Can you work these out from the drawing? Everything is in mm from the part's minimum corner. A direction names the side the tool comes from. Round coordinates to 2 decimals unless told otherwise and drop trailing zeros. Write each loop counter-clockwise with the first axis right and the second up, starting at its lowest first coordinate (ties: lowest second). Pieces come first, ordered by that corner, then holes. Notation, with made-up numbers: (-8, 61.5) - (27, 61.5) arc R11 ccw to (27, 81.5) - close; hole circle Ø10 at (66.25, 86). An arc over 180 degrees is marked (long way). Write each question's results on one line, items separated by ' | '. Start each with the question number.
(1) Please list where these lines run through material, in increasing order: line 1 (X direction, y = 1, z = 15); line 2 (Z direction, x = 15, y = 4.75); line 3 (Z direction, x = 25, y = 0.55). Write a range as [from, to].
(2) Thinking about a two-plate mould opening in Z: for the marked faces 1, 2 and 3, which applies, +Z half, -Z half, draft (parallel to the pull), parting line (faces both ways), or undercut?
(3) Imagine slicing it at B-B on y = 9.5. Write out the boundary of the cut face in (x, z).
(4) For P1, Ø5, axis at x = 15.5, z = 9, coming from the +Y side; P2, Ø4.5, axis at x = 25, z = 15, coming from the -Y side; P3, Ø1, axis at y = 8.5, z = 18.5, coming from the +X side; P4, Ø3, axis at x = 5, z = 15, coming from the -Y side, each with a flat end and sliding along its axis, tell me the tip position at first contact or that it passes through.
(5) Imagine slicing it at D-D on x = 10.5. Write out the boundary of the cut face in (y, z), then the cut area to 3 significant figures.
(6) Imagine slicing it at C-C on y = 2.75. Write out the boundary of the cut face in (x, z), then the cut area to 3 significant figures.
(7) Imagine slicing it at A-A on x = 15. Write out the boundary of the cut face in (y, z).
(8) On a 3-axis mill with a long thin cutter (end or side, diameter ignored), from which of +Z, -Z, +X, -X, +Y, -Y can I reach the whole of each face in a straight line? I mean the marked faces 4 and 5. Say none if no direction works.
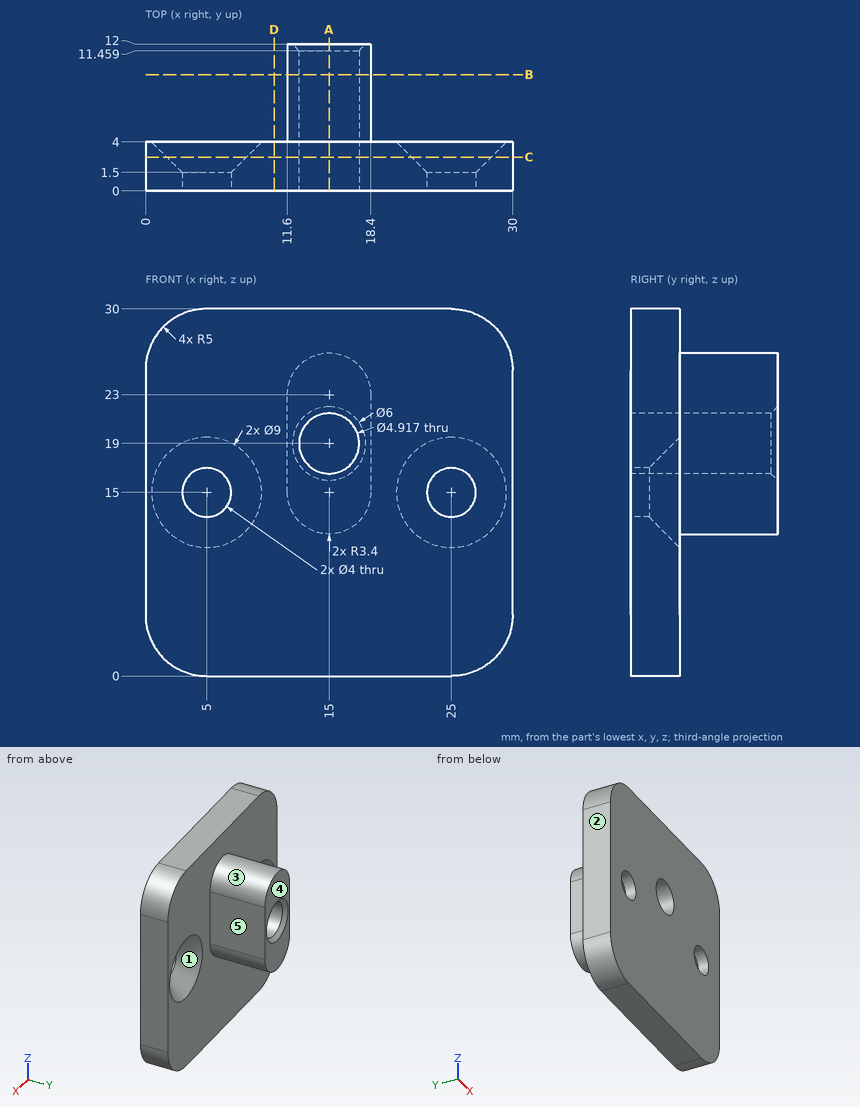
Response:
1) line 1: [0, 3], [7, 23], [27, 30] | line 2: [11.6, 16.54], [21.46, 26.4] | line 3: [0, 13], [17, 30]
2) face 1: undercut | face 2: draft | face 3: +Z half
3) outline: (11.6, 15) arc R3.4 ccw to (18.4, 15) - (18.4, 23) arc R3.4 ccw to (11.6, 23) - close; hole circle Ø4.92 at (15, 19)
4) P1: y = 4 | P2: y = 0 | P3: x = 18.4 | P4: through
5) outline: (0, 0) - (4, 0) - (4, 30) - (0, 30) - close | area: 120 mm²
6) outline: (0, 5) arc R5 ccw to (5, 0) - (25, 0) arc R5 ccw to (30, 5) - (30, 25) arc R5 ccw to (25, 30) - (5, 30) arc R5 ccw to (0, 25) - close; hole circle Ø6.5 at (5, 15); hole circle Ø4.92 at (15, 19); hole circle Ø6.5 at (25, 15) | area: 793 mm²
7) outline: (0, 0) - (4, 0) - (4, 11.6) - (12, 11.6) - (12, 16) - (11.46, 16.54) - (0, 16.54) - close; (0, 21.46) - (11.46, 21.46) - (12, 22) - (12, 26.4) - (4, 26.4) - (4, 30) - (0, 30) - close
8) face 4: +Z, -Z, +X, -X, +Y | face 5: +Z, -Z, +X, +Y
